Geometry: final body of the model. Coordinates: model frame, mm. Coordinates: 2 decimals unless noted, no trailing zeros. Write each loop counter-clockwise with the first axis right and the second up, starting at its lowest first coordinate (ties: lowest second). Pieces come first, ordered by that corner, then holes. Notation, with made-up numbers: (10, 3.25) -> (23, 3.25) arc R17 cw to (23, 33.25) -> close; hole circle Ø4 at (-22.5, -38.5). An arc over 180 degrees is marked (long way). One line per item, written item: value. Start each with the question number.
from build123d import *

# Parameters (mm, degrees)
SKETCH_W     = 40
SKETCH_H     = 40
SKETCH_R     = 1.75
PAD_DEPTH    = 10
FILLET_R     = 4
SKETCH001_R  = 19
POCKET_DEPTH = 10.001


with BuildPart() as part:
    # Sketch → Pad (new body)
    with BuildSketch(Plane.XY):
        Rectangle(SKETCH_W, SKETCH_H)
        with Locations((-16, 16)):
            Circle(SKETCH_R, mode=Mode.SUBTRACT)
        with Locations((16, 16)):
            Circle(SKETCH_R, mode=Mode.SUBTRACT)
        with Locations((16, -16)):
            Circle(SKETCH_R, mode=Mode.SUBTRACT)
        with Locations((-16, -16)):
            Circle(SKETCH_R, mode=Mode.SUBTRACT)
    extrude(amount=PAD_DEPTH)

    # Fillet
    fillet_edges = [part.edges().sort_by_distance(p)[0] for p in [
        (20, -20, 5),
        (-20, -20, 5),
        (20, 20, 5),
        (-20, 20, 5),
    ]]
    fillet(fillet_edges, radius=FILLET_R)

    # Sketch001 (on Face5 of Fillet) → Pocket (cut, through all)
    with BuildSketch(Plane.XY.offset(10)):
        Circle(SKETCH001_R)
    extrude(amount=-POCKET_DEPTH, mode=Mode.SUBTRACT)


solid = part.part
Q1. Line query: L1, parallel to Y at x = 14.5, z = 4.5; L2, parallel to Y at x = 16, z = 3.5. Output: solid intervals per line, ascending. Write a range as from..to.
Q2. Cut plane C-C on z = 0.5. Output: boundary loops of the cut face in (x, y), and give its area (3 significant figures).
Q3. Draft query along X for faces 1 (the cylindrical face through (-16.228, -14.265, 4.93)), 2 (the flat face through (20, 0, 5)), 3 (the cylindrical face through (-18.859, 18.797, 5.07)). Return one class per face: pulls with the +X half, pulls with the -X half, needs draft (parallel to the pull), parting line crosses it, or undercut.
Q4. Cut plane A-A on y = 0. Output: boundary loops of the cut face in (x, z), and give its area (3 significant figures).
Q5. Cut plane D-D on x = -15.5. Output: boundary loops of the cut face in (y, z).
Solution:
1. L1: -20..-16.9, -15.1..-12.28, 12.28..15.1, 16.9..20
1. L2: -20..-17.75, -14.25..-10.25, 10.25..14.25, 17.75..20
2. outline: (-20, -16) arc R4 ccw to (-16, -20) -> (16, -20) arc R4 ccw to (20, -16) -> (20, 16) arc R4 ccw to (16, 20) -> (-16, 20) arc R4 ccw to (-20, 16) -> close; hole circle Ø38 at (0, 0); hole circle Ø3.5 at (-16, -16); hole circle Ø3.5 at (-16, 16); hole circle Ø3.5 at (16, -16); hole circle Ø3.5 at (16, 16)
2. area: 414 mm²
3. face 1: undercut
3. face 2: pulls with the +X half
3. face 3: pulls with the -X half
4. outline: (-20, 0) -> (-19, 0) -> (-19, 10) -> (-20, 10) -> close; (19, 0) -> (20, 0) -> (20, 10) -> (19, 10) -> close
4. area: 20.0 mm²
5. outline: (-20, 0) -> (-17.68, 0) -> (-17.68, 10) -> (-20, 10) -> close; (-14.32, 0) -> (-10.99, 0) -> (-10.99, 10) -> (-14.32, 10) -> close; (10.99, 0) -> (14.32, 0) -> (14.32, 10) -> (10.99, 10) -> close; (17.68, 0) -> (20, 0) -> (20, 10) -> (17.68, 10) -> close
